Input: part model. Units: mm. Frame: model coordinates. A direction names the side the tool comes from. Give positions to 0.01 mm unless a question says otherwise; leave off trailing zeros. Loops run counter-clockwise (first coordinate to the right, second up) from the corner with the lowest first, then second, coordinate; pieces in that order, holes last. Notation, with made-up numbers: (-16.5, 25) - (-10.5, 25) arc R20 ccw to (-10.5, 53) - close; hole circle Ø9 at (-28.5, 33.25). An arc over 180 degrees is marked (long way). One line per item, written item: value.
from build123d import *

# Parameters (mm, degrees)
F1_DEPTH = 101.6
F2_W     = 103.886
F2_H     = 95.151683
F3_DEPTH = 22.86


with BuildPart() as f1:
    # F0 (on Front) → F1 (new body)
    with BuildSketch(Plane.XZ):
        Polygon((-55.959374, 25.4), (-55.959374, 0), (96.440626, 0), (96.440626, 51.377271), (92.084546, 51.377271), (92.084546, 25.4), align=None)
    extrude(amount=F1_DEPTH)

    # F2 (on face) → F3 (cut)
    with BuildSketch(Plane.XY.offset(25.4)):
        with Locations((-0.603251, -50.790785)):
            Rectangle(F2_W, F2_H)
    extrude(amount=-F3_DEPTH, mode=Mode.SUBTRACT)


solid = f1.part
Item 1: Access query for faces 1 (the face through (57, -47, 25.4)), 2 (the face through (-1, -98.367, 14)), 3 (the face through (96.441, -50, 25)). Directions: +Z, -Z, +X, -X, +Y, -Y. A direction counts if a zero-diameter tool reaches every point of the face in a straight line with its end or side. Return the directions, or none.
Verdict:
face 1: +Z, -X, +Y, -Y
face 2: +Z
face 3: +Z, -Z, +X, +Y, -Y
Item 2: Section C-C, the plane y = -36. Output: boundary loops of the cut face in (x, z), and give its area (3 significant figures).
Verdict:
outline: (-55.96, 0) - (96.44, 0) - (96.44, 51.38) - (92.08, 51.38) - (92.08, 25.4) - (51.34, 25.4) - (51.34, 2.54) - (-52.55, 2.54) - (-52.55, 25.4) - (-55.96, 25.4) - close
area: 1,610 mm^2
Item 3: Section D-D, the plane z = 43.5. Output: boundary loops of the cut face in (x, y).
Verdict:
outline: (92.08, -101.6) - (96.44, -101.6) - (96.44, 0) - (92.08, 0) - close
Item 4: Pin query (flat end, axial travel): P1, Ø1.5, axis at x = 78, y = -31, coming from the +Z side; P2, Ø6, axis at y = -12, z = 41, coming from the -X side; P3, Ø3, axis at x = 26, y = -68, coming from the +Z side. Return the tip coordinate at first contact, or that it passes through.
Verdict:
P1: stops at z = 25.4
P2: stops at x = 92.08
P3: stops at z = 2.54
Item 5: Material intervals for L1, parallel to X at y = -52, z = 20; L2, parallel to Y at x = -14, z = 8; L3, parallel to Z at x = 78.5, y = -55, sorted ascending.
Verdict:
L1: x = -55.96 to -52.55, 51.34 to 96.44
L2: y = -101.6 to -98.37, -3.21 to 0
L3: z = 0 to 25.4
Item 6: Section B-B, the plane x = 19. Output: boundary loops of the cut face in (y, z).
Verdict:
outline: (-101.6, 0) - (0, 0) - (0, 25.4) - (-3.21, 25.4) - (-3.21, 2.54) - (-98.37, 2.54) - (-98.37, 25.4) - (-101.6, 25.4) - close
Item 7: Section A-A, the plane z = 18. Output: boundary loops of the cut face in (x, y), and give its area (3 significant figures).
Verdict:
outline: (-55.96, -101.6) - (96.44, -101.6) - (96.44, 0) - (-55.96, 0) - close; hole (-52.55, -98.37) - (51.34, -98.37) - (51.34, -3.21) - (-52.55, -3.21) - close
area: 5,600 mm^2
Item 8: Draft query along Y for faces 4 (the face through (94, -50, 51.377)), 5 (the face through (19, -101.6, 15)), 6 (the face through (-1, -3.215, 14)). Return one class per face: pulls with the +Y half, pulls with the -Y half, needs draft (parallel to the pull), parting line crosses it, or undercut.
Verdict:
face 4: needs draft
face 5: pulls with the -Y half
face 6: undercut
